```python
from build123d import *

# Parameters (mm, degrees)
F0_W     = 147.32
F0_H     = 66.548
F1_DEPTH = 82.296
F2_W     = 66.548
F2_H     = 23.203082
F3_DEPTH = 124.968
F4_W     = 66.548
F4_H     = 41.148
F5_DEPTH = 124.968


with BuildPart() as f1:
    # F0 (on Top) → F1 (new body)
    with BuildSketch(Plane.XY):
        with Locations((-33.647868, -0.571987)):
            Rectangle(F0_W, F0_H)
    extrude(amount=F1_DEPTH)

    # F2 (on face) → F3 (cut)
    with BuildSketch(Plane.YZ.offset(40.012132)):
        with Locations((-0.571987, 11.601541)):
            Rectangle(F2_W, F2_H)
    extrude(amount=-F3_DEPTH, mode=Mode.SUBTRACT)

    # F4 (on face) → F5 (cut)
    with BuildSketch(Plane(origin=(-107.307868, 0, 0), x_dir=(0, -1, 0), z_dir=(-1, 0, 0))):
        with Locations((0.571987, 61.722)):
            Rectangle(F4_W, F4_H)
    extrude(amount=-F5_DEPTH, mode=Mode.SUBTRACT)


solid = f1.part
```
CAD build for the part. Positions are in the model's coordinates, mm. A direction names the side the tool comes from. Round coordinates to 2 decimals unless told otherwise and drop trailing zeros. Write each loop counter-clockwise with the first axis right and the second up, starting at its lowest first coordinate (ties: lowest second). Pieces come first, ordered by that corner, then holes.
Item 1: Band-saw the part on A-A on y = -5.5. Write the cut outline in (x, z).
Filled in:
outline: (-107.31, 0) - (-84.96, 0) - (-84.96, 23.2) - (40.01, 23.2) - (40.01, 82.3) - (17.66, 82.3) - (17.66, 41.15) - (-107.31, 41.15) - close
Item 2: Drill centre lines: L1, parallel to X at y = -1.5, z = 15; L2, parallel to Z at x = -43, y = -26.5; L3, parallel to X at y = -31, z = 42.5. Where is each one in solid material? Low to high.
Filled in:
L1: x = -107.31 to -84.96
L2: z = 23.2 to 41.15
L3: x = 17.66 to 40.01
Item 3: Band-saw the part on B-B on x = -83. Write the cut outline in (y, z), then the cut area to 3 significant figures.
Filled in:
outline: (-33.85, 23.2) - (32.7, 23.2) - (32.7, 41.15) - (-33.85, 41.15) - close
area: 1,190 mm2
Item 4: Tool access for faces 1 (the flat face through (-46, 0, 41.148)), 2 (the flat face through (-84.956, -1, 12)), 3 (the flat face through (40.012, -1, 52)): list every direction of +Z, -Z, +X, -X, +Y, -Y with a clear straight run to the whole face (end or side of a thin tool).
Filled in:
face 1: +Z, -X, +Y, -Y
face 2: -Z, +X, +Y, -Y
face 3: +Z, -Z, +X, +Y, -Y
Item 5: Drop flat-ended pins along their axis: pin 1 Ø12.5 at (y, z) = (11.5, 71.5) entering from -X; pin 2 Ø20 at (x, y) = (-68, -6.5) entering from +Z; pin 3 Ø1.5 at (x, y) = (-76.5, -4.5) entering from -Z. Give the stop position or say it passes through.
Filled in:
pin 1: stops at x = 17.66
pin 2: stops at z = 41.15
pin 3: stops at z = 23.2
Item 6: Band-saw the part on C-C on z = 18.5. Write the cut outline in (x, y).
Filled in:
outline: (-107.31, -33.85) - (-84.96, -33.85) - (-84.96, 32.7) - (-107.31, 32.7) - close
